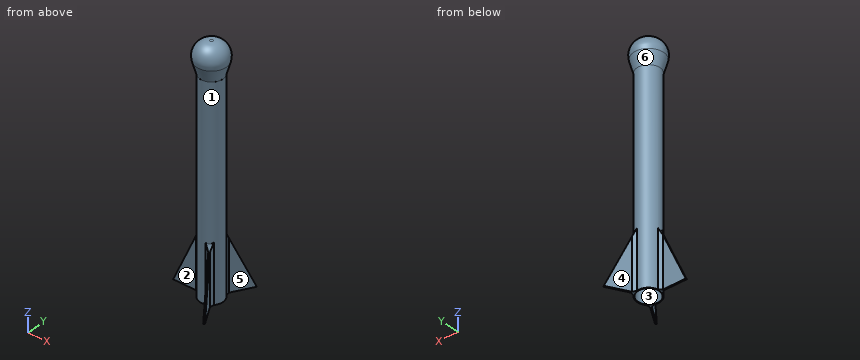
from build123d import *

# Parameters (mm, degrees)
SKETCH_R           = 8.9
PAD_DEPTH          = 160
SKETCH001_R        = 8.3
POCKET_DEPTH       = 158
PAD001_DEPTH       = 1
POLARPATTERN_COUNT = 3
CHAMFER_SIZE       = 2


with BuildPart() as part:
    # Sketch → Pad (new body)
    with BuildSketch(Plane.XY):
        Circle(SKETCH_R)
    extrude(amount=PAD_DEPTH)

    # Sketch001 (on Face2 of Pad) → Pocket (cut)
    with BuildSketch(Plane(origin=(0, 0, 0), x_dir=(1, 0, 0), z_dir=(0, 0, -1))):
        Circle(SKETCH001_R)
    extrude(amount=-POCKET_DEPTH, mode=Mode.SUBTRACT)

    # Sketch002 → Pad001 (join)
    with BuildSketch(Plane.XZ):
        Polygon((-8.35, 45), (-28.35, 0), (-8.35, 0), align=None)
    pad001 = extrude(amount=PAD001_DEPTH)

    # PolarPattern: Pad001 ×3 about axis
    polarpattern_axis = Axis((0, 0, 0), (0, 0, 1))
    for i in range(1, POLARPATTERN_COUNT):
        add(pad001.rotate(polarpattern_axis, i * 360 / POLARPATTERN_COUNT))

    # Sketch003 → Revolution (revolve)
    with BuildSketch(Plane.XZ):
        with BuildLine():
            Line((-1.135739, 183.616416), (0, 183.616416))
            Line((0, 183.616416), (0, 159.771789))
            Line((0, 159.771789), (-8.8, 159.771789))
            Line((-8.8, 159.771789), (-11.616332, 169.779203))
            ThreePointArc((-1.135739, 183.616416), (-9.8149, 179.302476), (-11.616332, 169.779203))
        make_face()
    revolve(axis=Axis((0, 0, 0), (0, 0, 1)))

    # Chamfer
    chamfer_edges = [part.edges().sort_by_distance(p)[0] for p in [
        (4.45, 7.707626, 21.88125),
        (5.287846, -7.158818, 21.944653),
        (4.45, -7.707626, 21.88125),
        (-8.843642, -1, 21.944653),
        (-8.9, 0, 21.88125),
        (3.555795, 8.158818, 21.944653),
    ]]
    chamfer(chamfer_edges, length=CHAMFER_SIZE)


solid = part.part
Read the model definition and answer for the solid it produces. Units are mm, in the model's axes. Face numbers are marked on the shaded views. A direction names the side the tool comes from. Round coordinates to 2 decimals unless told otherwise and drop trailing zeros. Loops run counter-clockwise (first coordinate to the right, second up) from the corner with the lowest first, then second, coordinate; pieces in that order, holes last.
Q1. Section B-B on y = -20 is taken. Write down the section's boundary in (x, z), and give its area (3 significant figures).
Q2. Which of the six approach directions +Z, -Z, +X, -X, +Y, -Y give full straight-line access (tool end or side, diameter ignored) to the marked faces 1, 2 and 3?
Q3. Section A-A on z = 24 is taken. Write down the section's boundary in (x, y).
Q4. Section D-D on x = -19 is taken. Write down the section's boundary in (y, z), and give its area (3 significant figures).
Q5. Consider probe 1 along Y at (x, z) = (0, 81); probe 2 along Y at (x, z) = (-5, 64). Determine where each line is inside the solid, lowest interval first.
Q6. Each of these flat-tipped pins is pushed along its axis until it touches: pin 1 (10 mm diameter, centred on y = -15.5, z = 40.5, fed in from +X); pin 2 (4 mm diameter, centred on x = 8.5, z = 96, fed in from -Y); pin 3 (4 mm diameter, centred on x = -23, y = 0, fed in from +Z); pin 4 (10 mm diameter, centred on y = 12.5, z = 86.5, fed in from -X). Where does it stop, or does it pass through?
Q7. Section C-C on z = 100.5 is taken. Write down the section's boundary in (x, y).
Q8. Determine the mould class of the marked faces 4, 5 and 6 for opening direction Y: released by +Y, released by -Y, zero draft, split by the parting line, or undercut.
Output:
1. outline: (11.55, 0) - (12.7, 0) - (12.7, 10.53) - (11.55, 11.83) - close
1. area: 12.9 mm2
2. face 1: none
2. face 2: -Z, -X, -Y
2. face 3: -Z
3. outline: (-17.68, -1) - (-10.84, -1) - (-8.4, -2.95) arc R8.9 ccw to (2.62, -8.51) - (5.45, -9.44) - (8.84, -15.31) - (9.71, -14.81) - (6.29, -8.89) - (6.75, -5.8) arc R8.9 ccw to (6.06, 6.52) - (5.45, 9.44) - (8.84, 15.31) - (7.98, 15.81) - (4.56, 9.89) - (1.64, 8.75) arc R8.9 ccw to (-8.68, 1.99) - (-10.9, 0) - (-17.68, 0) - close; hole circle Ø16.6 at (0, 0)
4. outline: (-1, 0) - (0, 0) - (0, 21.04) - (-1, 21.04) - close
4. area: 21.0 mm2
5. probe 1: y = -8.9 to -8.3, 8.3 to 8.9
5. probe 2: y = -7.36 to -6.62, 6.62 to 7.36
6. pin 1: passes through
6. pin 2: stops at y = -6.08
6. pin 3: stops at z = 16.54
6. pin 4: stops at x = -4.79
7. outline: circle Ø17.8 at (0, 0); hole circle Ø16.6 at (0, 0)
8. face 4: released by +Y
8. face 5: undercut
8. face 6: split by the parting line
